CAD build for the part. Positions are in the model's coordinates, mm. A direction names the side the tool comes from. Coordinates: 2 decimals unless noted, no trailing zeros. Loops run counter-clockwise (first coordinate to the right, second up) from the corner with the lowest first, then second, coordinate; pieces in that order, holes last.
1) Which spindle directions (+Z, -Z, +X, -X, +Y, -Y) get a long thin tool onto all of the face, cutting with end or side? Do faces 4 (the flat face through (-179, -4.826, -94)), 5 (the flat face through (-91.44, -2, -153)), 6 (the flat face through (-87, -6.096, -43)). Say none if no direction does.
2) Wall check: line 1 along X through (y, z) = (-4.5, -38.1) (1 decimal); line 2 along X through (y, z) = (-2.75, -40.5); line 3 along Z through (x, y) = (-120, -5.25). Give the ranges that are in metal, low to high.
3) Saw through at C-C, the plane x = -134. Write the cut outline in (y, z), and give its area (3 significant figures).
4) Saw through at A-A, the plane x = -40.64. Write the cut outline in (y, z) (3 decimals).
5) Saw through at B-B, the plane z = -38.1. Write the cut outline in (x, y) (1 decimal).
6) Two-plate mould, pull along X, no slides. Class faces 1 (the flat face through (-148, 0, -70)), 2 (the cylindrical face through (-38.494, -3.005, -40.44)), 3 (the flat face through (-203.2, -3, -90)): +X half, -X half, draft (parallel to the pull), parting line (faces both ways), or undercut.
7) Saw through at D-D, the plane z = -60. Write the cut outline in (x, y).
8) Pin check, flat tips, straight feed: pin 1 Ø2.5 at (y, z) = (-1, -101.5) entering from +X; pin 2 Ø0.8 at (y, z) = (-3.5, -82.5) entering from +X. Stop position of each tip, or through.
```python
from build123d import *

# Parameters (mm, degrees)
SKETCH1_R           = 3.175
BOSS_EXTRUDE1_DEPTH = 6.096
SKETCH2_W           = 91.44
SKETCH2_H           = 152.4
CUT_EXTRUDE1_DEPTH  = 1.27
CUT_EXTRUDE2_DEPTH  = 3.81


with BuildPart() as part:
    # Sketch1 → Boss-Extrude1 (new body)
    with BuildSketch(Plane(origin=(0, 0, 0), x_dir=(1, 0, 0), z_dir=(0, 1, 0))):
        Polygon((0, 50.8), (-91.44, 50.8), (-91.44, 63.5), (-142.24, 63.5), (-142.24, 114.3), (-91.44, 114.3), (-91.44, 177.8), (-203.2, 177.8), (-203.2, 0), (0, 0), align=None)
        with Locations(Location((-15.24, 38.1, 0), (0, 0, 270))):  # turned: the seam where the file's is
            Circle(SKETCH1_R, mode=Mode.SUBTRACT)
        with Locations(Location((-40.64, 38.1, 0), (0, 0, 270))):  # turned: the seam where the file's is
            Circle(SKETCH1_R, mode=Mode.SUBTRACT)
        with Locations(Location((-40.64, 12.7, 0), (0, 0, 270))):  # turned: the seam where the file's is
            Circle(SKETCH1_R, mode=Mode.SUBTRACT)
        with Locations(Location((-15.200835983, 12.7, 0), (0, 0, 270))):  # turned: the seam where the file's is
            Circle(SKETCH1_R, mode=Mode.SUBTRACT)
    extrude(amount=-BOSS_EXTRUDE1_DEPTH)

    # Sketch2 → Cut-Extrude1 (cut)
    with BuildSketch(Plane.XZ.offset(6.096)):
        with Locations((-144.78, -88.9)):
            Rectangle(SKETCH2_W, SKETCH2_H)
    extrude(amount=-CUT_EXTRUDE1_DEPTH, mode=Mode.SUBTRACT)

    # Sketch3 → Cut-Extrude2 (cut)
    with BuildSketch(Plane.XZ.offset(6.096)):
        Polygon((-91.44, -50.8), (-94.060496217, -50.8), (-94.060496217, -25.4), (-177.8, -25.4), (-177.8, -152.4), (-91.44, -152.4), align=None)
    extrude(amount=-CUT_EXTRUDE2_DEPTH, mode=Mode.SUBTRACT)


solid = part.part
```
Data:
1. face 4: -Y
1. face 5: -Z, +X, +Y, -Y
1. face 6: +Z, -Z, +X, -X, -Y
2. line 1: x = -203.2 to -177.8, -94.1 to -43.8, -37.5 to -18.4, -12.1 to 0
2. line 2: x = -203.2 to -177.8, -94.06 to -42.72, -38.56 to -17.32, -13.16 to 0
2. line 3: z = -177.8 to -165.1, -12.7 to 0
3. outline: (-6.1, -177.8) - (0, -177.8) - (0, -114.3) - (-2.29, -114.3) - (-2.29, -152.4) - (-4.83, -152.4) - (-4.83, -165.1) - (-6.1, -165.1) - close; (-6.1, -12.7) - (-4.83, -12.7) - (-4.83, -25.4) - (-2.29, -25.4) - (-2.29, -63.5) - (0, -63.5) - (0, 0) - (-6.1, 0) - close
3. area: 452 mm2
4. outline: (-6.096, -50.8) - (0, -50.8) - (0, -41.275) - (-6.096, -41.275) - close; (-6.096, -34.925) - (0, -34.925) - (0, -15.875) - (-6.096, -15.875) - close; (-6.096, -9.525) - (0, -9.525) - (0, 0) - (-6.096, 0) - close
5. outline: (-203.2, -6.1) - (-190.5, -6.1) - (-190.5, -4.8) - (-177.8, -4.8) - (-177.8, -2.3) - (-94.1, -2.3) - (-94.1, -6.1) - (-43.8, -6.1) - (-43.8, 0) - (-203.2, 0) - close; (-37.5, -6.1) - (-18.4, -6.1) - (-18.4, 0) - (-37.5, 0) - close; (-12.1, -6.1) - (0, -6.1) - (0, 0) - (-12.1, 0) - close
6. face 1: draft
6. face 2: undercut
6. face 3: -X half
7. outline: (-203.2, -6.1) - (-190.5, -6.1) - (-190.5, -4.83) - (-177.8, -4.83) - (-177.8, -2.29) - (-91.44, -2.29) - (-91.44, 0) - (-203.2, 0) - close
8. pin 1: stops at x = -142.24
8. pin 2: stops at x = -177.8
